Read the model definition and answer for the solid it produces. Units are mm, in the model's axes. A direction names the side the tool comes from. Coordinates: 2 decimals unless noted, no trailing zeros. Write each loop counter-clockwise with the first axis right and the second up, starting at its lowest first coordinate (ties: lowest second). Pieces come first, ordered by that corner, then holes. Notation, with made-up numbers: (85, 84.25) - (137, 84.25) arc R17 cw to (137, 114.25) - close; hole circle Ø11 at (-27, 67.5). An arc over 180 degrees is marked (long way). Return JSON: item names as keys, results as strings.
```python
from build123d import *


with BuildPart() as part:
    # Эскиз1 → Повернуть1 (revolve)
    with BuildSketch(Plane.XY):
        with BuildLine():
            Line((0, 0), (10, 0))
            ThreePointArc((10, 0), (80.710678119, 29.289321881), (110, 100))
            Line((110, 100), (110, 1507.617384372))
            ThreePointArc((110, 1507.617384372), (104.090062317, 1531.198444671), (87.757343806, 1549.205001097))
            Line((87.757343806, 1549.205001097), (43.961595612, 1578.436145741))
            ThreePointArc((43.961595612, 1578.436145741), (39.061780059, 1583.838112668), (37.288798754, 1590.912430758))
            Line((37.288798754, 1590.912430758), (37.288798754, 1614.158761672))
            ThreePointArc((37.288798754, 1614.158761672), (32.895400472, 1624.76536339), (22.288798754, 1629.158761672))
            Line((22.288798754, 1629.158761672), (0, 1629.158761672))
            Line((0, 1629.158761672), (0, 0))
        make_face()
    revolve(axis=Axis((0, 1553.075867376, 0), (0, -1, 0)))


solid = part.part
```
(1) Straight lines are drawn through the part: line 1 (Z direction, x = 5, y = 722.5); line 2 (X direction, y = 527.5, z = -6.5); line 3 (Z direction, x = 7, y = 1116.5). For each, find the intervals that lie inside material, in ascending order. Write a range as from..to.
Answer:
{"line 1": "-109.89..109.89", "line 2": "-109.81..109.81", "line 3": "-109.78..109.78"}
(2) A cutting plane is placed at A-A (y = 1071). Determine the outline of the cut face in (x, z).
Answer:
{"outline": "circle Ø220 at (0, 0)"}
(3) Flat-ended cylindrical pins translate along their axes: P1, Ø3, axis at y = 1147.5, z = 45, coming from the +X side; P2, Ø12, axis at x = -64, z = 73, coming from the -Y side; P3, Ø2, axis at x = -41, z = -66, coming from the +Y side. Find the tip coordinate at first contact, or state that the pin passes through.
Answer:
{"P1": "x = 101.03", "P2": "y = 41.47", "P3": "y = 1556.59"}
(4) Which of the six approach directions +Z, -Z, +X, -X, +Y, -Y give full straight-line access (tool end or side, diameter ignored) to faces 1 (the face through (-29.59, 1602.7, -22.69)), 2 (the face through (0, 1629.159, 0))?
Answer:
{"face 1": "+Y", "face 2": "+Z, -Z, +X, -X, +Y"}
